Geometry: final body of the model. Coordinates: model frame, mm. Round coordinates to 2 decimals unless told otherwise and drop trailing zeros. Loops run counter-clockwise (first coordinate to the right, second up) from the corner with the lowest first, then second, coordinate; pieces in that order, holes last. Notation, with made-up numbers: (66, -16.5) - (108, -16.5) arc R26 ccw to (108, 14.5) - close; hole circle Ø11 at (-31, 1.25). An arc over 180 degrees is marked (long way). Answer as CSV lines item,"result".
from build123d import *

# Parameters (mm, degrees)
BOSS_EXTRUDE1_DEPTH = 10
M6_TAPPED_HOLE_D    = 5


with BuildPart() as part:
    # Sketch1 → Boss-Extrude1 (new body)
    with BuildSketch(Plane.XY):
        with BuildLine():
            Line((-120, -760), (-200, -760))
            ThreePointArc((-200, -760), (-203.535533906, -758.535533906), (-205, -755))
            Line((-205, -755), (-205, -5))
            ThreePointArc((-205, -5), (-203.535533906, -1.464466094), (-200, 0))
            Line((-200, 0), (40, 0))
            ThreePointArc((40, 0), (43.535533906, -1.464466094), (45, -5))
            Line((45, -5), (45, -755))
            ThreePointArc((45, -755), (43.535533906, -758.535533906), (40, -760))
            Line((40, -760), (-40, -760))
            ThreePointArc((-40, -760), (-43.535533906, -758.535533906), (-45, -755))
            Line((-45, -755), (-45, -155))
            ThreePointArc((-45, -155), (-46.464466094, -151.464466094), (-50, -150))
            Line((-50, -150), (-110, -150))
            ThreePointArc((-110, -150), (-113.535533906, -151.464466094), (-115, -155))
            Line((-115, -155), (-115, -755))
            ThreePointArc((-115, -755), (-116.464466094, -758.535533906), (-120, -760))
        make_face()
    extrude(amount=BOSS_EXTRUDE1_DEPTH)

    # M6 Tapped Hole (through all)
    with Locations(Plane(origin=(479.845790405, 700.886073068, 20), x_dir=(-1, 0, 0), z_dir=(0, 0, 1))):
        with Locations((514.845790405, 897.471608895), (537.845790405, 897.471608895), (581.845790405, 897.471608895), (604.845790405, 897.471608895), (514.845790405, 1450.886073068), (514.845790405, 1412.886073068), (537.845790405, 1453.886073068), (537.845790405, 1409.886073068), (581.845790405, 1453.886073068), (581.845790405, 1409.886073068), (604.845790405, 1450.886073068), (604.845790405, 1412.886073068), (514.845790405, 1431.886073068), (537.845790405, 1431.886073068), (581.845790405, 1431.886073068), (604.845790405, 1431.886073068)):
            Hole(M6_TAPPED_HOLE_D / 2)


solid = part.part
(1) Section B-B (x = -56.5). Output: boundary loops of the cut face in (y, z), and give its area (3 significant figures).
Findings below:
outline,"(-150, 0) - (0, 0) - (0, 10) - (-150, 10) - close"
area,"1,500 mm2"
(2) Material intervals for line 1 along X through (y, z) = (-712, 4.25); line 2 along Y through (x, z) = (-35, 3.25); line 3 along X through (y, z) = (-214, 6), sorted ascending.
Findings below:
line 1,"-205 to -127.5, -122.5 to -115, -45 to -37.5, -32.5 to 45"
line 2,"-760 to -752.5, -747.5 to -733.5, -728.5 to -714.5, -709.5 to -199.09, -194.09 to 0"
line 3,"-205 to -115, -45 to 45"
(3) Pin query (flat end, axial travel): P1, Ø5, axis at x = -83, z = 5, coming from the -Y side. Return the tip coordinate at first contact, or that it passes through.
Findings below:
P1,"y = -150"
(4) Section A-A (y = -564). Output: boundary loops of the cut face in (x, z), and give its area (3 significant figures).
Findings below:
outline,"(-205, 0) - (-115, 0) - (-115, 10) - (-205, 10) - close; (-45, 0) - (45, 0) - (45, 10) - (-45, 10) - close"
area,"1,800 mm2"
(5) Section C-C (z = 6). Give the number of separate pieces and of enclosed holes in the cut face, and give its area (3 significant figures).
Findings below:
separate pieces,"1"
enclosed holes,"8"
area,"147,000 mm2"
